Autodesk Inventor part; units mm, degrees
ref_plane "YZ Plane" through (0, 0, 0) normal (1, 0, 0) x (0, 1, 0)
ref_plane "XZ Plane" through (0, 0, 0) normal (0, 1, 0) x (-1, 0, 0)
ref_plane "XY Plane" through (0, 0, 0) normal (0, 0, 1) x (1, 0, 0)
sketch "Sketch1" plane through (0, 0, 0) normal (0, 0, 1) x (1, 0, 0)
  circle A0 centre (0, 0) radius 336.55
  circle A1 centre (0, 0) radius 368.3
  dimension "d0" = 673.1
  dimension "d1" = 736.6
extrude "Extrusion1" add sketch "Sketch1" along normal blind 304.8
sketch "Sketch2" plane through (0, 0, 304.8) normal (0, 0, 1) x (1, 0, 0)
  circle A0 centre (0, 0) radius 368.3
  circle A1 centre (0, 0) radius 371.221
  circle A2 centre (0, 0) radius 374.396
  dimension "d4" = 742.442
  dimension "d5" = 748.792
extrude "Extrusion2" add sketch "Sketch2" against normal blind 50.8 contours A1
extrude "Extrusion3" add sketch "Sketch2" against normal blind 25.4 contours A2
chamfer "Chamfer1" distance 2.921 angle 45 1 edges at (-368.3, 0, 254)
sketch "Sketch3" plane through (0, 0, 0) normal (0, 0, -1) x (-1, 0, 0)
  circle A0 centre (0, 0) radius 355.346
  circle A1 centre (0, 0) radius 336.55
  dimension "d13" = 710.692
extrude "Extrusion4" add sketch "Sketch3" along normal blind 12.7
fillet "Fillet1" radius 0.7937 2 edges at (355.346, 0, 0) (-371.221, 0, 279.4)
chamfer "Chamfer2" distance 0.7937 angle 45 1 edges at (355.346, 0, -12.7)
chamfer "Chamfer3" distance 0.7937 angle 45 1 edges at (-374.396, 0, 279.4)
sketch "Sketch4" plane through (0, 0, 0) normal (1, 0, 0) x (0, 1, 0)
  line L0 (371.221, 278.6063) -> (371.221, 254) construction
  line L1 (-374.396, 304.8) -> (374.396, 304.8) construction
  line L2 (371.221, 273.05) -> (369.4409, 271.2699)
  arc A0 (369.4409, 271.2699) -> (368.046, 267.9023) centre (372.8085, 267.9023) ccw
  line L3 (368.046, 267.9023) -> (368.046, 267.0852)
  arc A1 (368.046, 267.0852) -> (369.4409, 263.7176) centre (372.8085, 267.0852) ccw
  line L4 (369.4409, 263.7176) -> (371.221, 261.9375)
  line L5 (371.221, 261.9375) -> (371.221, 273.05)
  line L6 (0, -76.2) -> (0, 368.3)
  point P0 (0, 0)
  dimension "d23" = 11.1125
  dimension "d24" = 3.175
  dimension "d25" = 4.7625
  dimension "d26" = 31.75
  dimension "d27" = 45
revolve "Revolution1" cut sketch "Sketch4" angle 360 about axis through (0, 0, -10) along (0, 0, 1)
equation "\"d10\" = -0.5 * d1 + 0.5 * d4"
properties part number "A1-19037-100-06 HCWI liner - pup" material "Iron, HCWI"
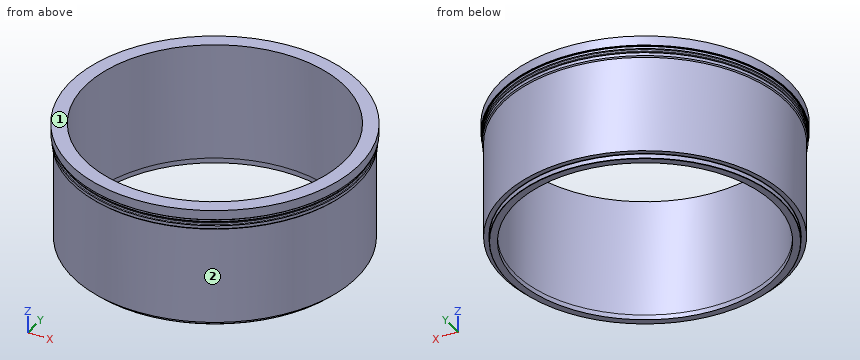
For this review, take the finished solid that the model builds, in its own axes (mm). Face numbers are marked on the shaded views. A direction names the side the tool comes from. Give positions to 0.01 mm unless a question says otherwise; leave off trailing zeros. Write each loop counter-clockwise with the first axis right and the second up, starting at its lowest first coordinate (ties: lowest second). Pieces come first, ordered by that corner, then holes.
Item 1: Insertion check: P1, Ø10, axis at x = -162.5, z = 97, coming from the +Y side; P2, Ø3, axis at y = -49, z = 263.5, coming from the +X side; P3, Ø10, axis at y = -274, z = 232, coming from the +X side. Each pin has a flat end and moves straight along its axis. Give the tip position at first contact, or say it passes through.
Item 2: Take a section at A-A (z = 187.5). Give the boundary of the cut face in (x, y), and give its area (3 significant figures).
Item 3: Wall thickness on probe 1 along Y at (x, z) = (0, -9.75); probe 2 along Y at (x, z) = (0, 152); probe 3 along Z at (x, y) = (282, -246): over which ranges is each line inside the solid? List them lowest first.
Item 4: Machinability: for the marked faces 1 and 2, which of the approach directions +Z, -Z, +X, -X, +Y, -Y give a long, thin tool a straight path to every point of the face, cutting with its end or side? Answer none if there is none.
Established:
1. P1: stops at y = 332.92
1. P2: stops at x = 367.92
1. P3: stops at x = 251.56
2. outline: circle Ø736.6 at (0, 0); hole circle Ø673.1 at (0, 0)
2. area: 70,300 mm2
3. probe 1: y = -355.35 to -336.55, 336.55 to 355.35
3. probe 2: y = -368.3 to -336.55, 336.55 to 368.3
3. probe 3: z = 280.02 to 304.8
4. face 1: +Z, +X, -X, +Y, -Y
4. face 2: -Z
